Input: part model. Units: mm. Frame: model coordinates. A direction names the side the tool comes from. Give positions to 0.01 mm unless a question says otherwise; leave off trailing zeros. Loops run counter-clockwise (first coordinate to the right, second up) from the corner with the lowest first, then second, coordinate; pieces in that order, holes last. Notation, with made-up numbers: M -1,-11 L 8,-11 A19 ccw 8,5 Z; hole C 48.5,-14 d11. An arc over 180 degrees is marked long. Use a Markdown table: item, result. Add a question column.
Autodesk Inventor part; units mm, degrees
ref_plane "YZ Plane" through (0, 0, 0) normal (1, 0, 0) x (0, 1, 0)
ref_plane "XZ Plane" through (0, 0, 0) normal (0, 1, 0) x (-1, 0, 0)
ref_plane "XY Plane" through (0, 0, 0) normal (0, 0, 1) x (1, 0, 0)
sketch "Skizze1" plane through (0, 0, 0) normal (1, 0, 0) x (0, 1, 0)
  circle A0 centre (0, 0) radius 40
  circle A1 centre (0, 0) radius 108
  dimension "d0" = 216
  dimension "d1" = 80
extrude "Extrusion1" add sketch "Skizze1" along normal blind 15
sketch "Skizze2" plane through (15, 0, 0) normal (1, 0, 0) x (0, 0, -1)
  circle A0 centre (0, 0) radius 40
  circle A1 centre (0, 0) radius 50
  dimension "d4" = 100
extrude "Extrusion2" add sketch "Skizze2" along normal blind 985
fillet "Rundung1" radius 10 1 edges at (15, 0, 50)
sketch "Skizze3" plane through (15, 0, 0) normal (1, 0, 0) x (0, 0, -1)
  circle A0 centre (0, -85) radius 10 construction
  line L0 (0, -95) -> (-8.7647, -89.8146)
  line L1 (-8.7647, -80.1854) -> (0, -75)
  line L2 (0, -75) -> (8.7647, -80.1854)
  line L3 (8.7647, -80.1854) -> (8.7647, -89.8146)
  line L4 (0, -95) -> (8.7647, -89.8146)
  line L5 (-8.7647, -80.1854) -> (-8.7647, -89.8146)
  point P0 (0, 0)
  dimension "d8" = 20
  dimension "d9" = 85
extrude "Extrusion3" add sketch "Skizze3" along normal blind 10
sketch "Skizze4" plane through (25, 0, 0) normal (1, 0, 0) x (0, 0, -1)
  circle A0 centre (0, -85) radius 5
  point P0 (0, 0)
  dimension "d12" = 10
extrude "Extrusion4" add sketch "Skizze4" along normal blind 10
pattern_circular "Runde Anordnung1" count 6 over 360 about axis through (-10, 0, 0) along (1, 0, 0) of "Extrusion3", "Extrusion4"
mirror "Spiegeln1" about plane through (1000, 0, 0) normal (1, 0, 0) of "Extrusion3", "Extrusion4", "Runde Anordnung1", "Extrusion2", "Extrusion1", "Rundung1"
properties part number "DN80-2m"
1) Pull-direction query (Y, two-part tool) for faces 3 (the flat face through (1985, -46, -46)), 4 (the flat face through (2000, -46, 2)), 5 (the cylindrical face through (7.395, -23.412, 105.432)); classes: pulls with the +Y half, pulls with the -Y half, needs draft (parallel to the pull), parting line crosses it, or undercut.
2) Contact query for flat-ended pins moving along their axis: P1, Ø5, axis at y = 40.5, z = -75, coming from the -X side; P2, Ø3, axis at x = 1980, y = 87, coming from the +Z side; P3, Ø10.5, axis at x = 1979.5, y = 86, coming from the -Z side; P4, Ø5, axis at x = 1421, z = -48, coming from the -Y side. Output: stop coordinate, or through.
3) Ray query, line 1 (X direction, y = 96, z = -10.5); line 2 (Z direction, x = 908, y = -2); line 3 (Z direction, x = 1320, y = 5). Return the intervals inside material, ascending. Write a range as [from, to].
4) Section query B-B, the plane x = 863. Return the cut outline in (y, z), and give its area (3 significant figures).
5) Section query A-A, the plane y = 0. Return the cut outline in (x, z).
6) Reachability of faces 1 (the flat face through (0, 46, 2)), 2 (the flat face through (15, 46, -46)) from +Z, -Z, +X, -X, +Y, -Y: full face, straight path, thin tool, end or side. Return the list, or none.
Entries:
| question | item | result |
|---|---|---|
| 1 | face 3 | undercut |
| 1 | face 4 | needs draft |
| 1 | face 5 | parting line crosses it |
| 2 | P1 | stops at x = 0 |
| 2 | P2 | stops at z = 8.76 |
| 2 | P3 | stops at z = -8.76 |
| 2 | P4 | stops at y = -20.73 |
| 3 | line 1 | x = [0, 15], [1985, 2000] |
| 3 | line 2 | z = [-49.96, -39.95], [39.95, 49.96] |
| 3 | line 3 | z = [-49.75, -39.69], [39.69, 49.75] |
| 4 | outline | C 0,0 d100; hole C 0,0 d80 |
| 4 | area | 2,830 mm² |
| 5 | outline | M 0,-108 L 15,-108 L 15,-60 A10 cw 25,-50 L 1975,-50 A10 cw 1985,-60 L 1985,-108 L 2000,-108 L 2000,-40 L 0,-40 Z; M 0,40 L 2000,40 L 2000,108 L 1985,108 L 1985,60 A10 cw 1975,50 L 25,50 A10 cw 15,60 L 15,108 L 0,108 Z |
| 6 | face 1 | +Z, -Z, -X, +Y, -Y |
| 6 | face 2 | none |
